Here's how the part is built. I have some questions about the finished solid (model axes, mm). Face numbers are marked on the shaded views. A direction names the side the tool comes from. Round coordinates to 2 decimals unless told otherwise and drop trailing zeros. Write each loop counter-clockwise with the first axis right and the second up, starting at its lowest first coordinate (ties: lowest second). Pieces come first, ordered by that corner, then holes. Notation, with made-up numbers: (73.25, 47) -> (107.25, 47) arc R24 ccw to (107.25, 71) -> close; hole circle Ø11 at (-29, 84.5). An arc over 180 degrees is marked (long way). Answer in a Markdown table with one row per item.
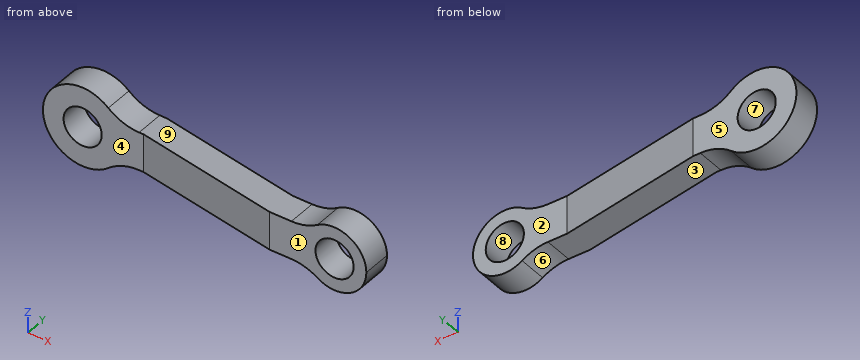
from build123d import *

# Parameters (mm, degrees)
F0_R     = 6
F1_DEPTH = 25
F3_DEPTH = 12.5
F4_R     = 15


with BuildPart() as f1:
    # F0 (on Front) → F1 (new body)
    with BuildSketch(Plane.XZ):
        with BuildLine():
            ThreePointArc((10.965856, -6), (12.110392, -3.096514), (12.5, 0))
            ThreePointArc((12.5, 0), (12.110392, 3.096514), (10.965856, 6))
            ThreePointArc((10.965856, 6), (-12.5, 0), (10.965856, -6))
        make_face()
        Circle(F0_R, mode=Mode.SUBTRACT)
        with BuildLine():
            ThreePointArc((10.965856, 6), (12.110392, 3.096514), (12.5, 0))
            ThreePointArc((12.5, 0), (12.110392, -3.096514), (10.965856, -6))
            Line((10.965856, -6), (77, -6))
            ThreePointArc((77, -6), (75, 0), (77, 6))
            Line((77, 6), (10.965856, 6))
        make_face()
        with BuildLine():
            ThreePointArc((95, 0), (88.162278, 9.486833), (77, 6))
            ThreePointArc((77, 6), (75, 0), (77, -6))
            ThreePointArc((77, -6), (88.162278, -9.486833), (95, 0))
        make_face()
        with Locations((85, 0)):
            Circle(F0_R, mode=Mode.SUBTRACT)
    extrude(amount=F1_DEPTH)

    # F2 (on Top) → F3 (intersect, symmetric)
    with BuildSketch(Plane.XY):
        Polygon((0, 0), (-12.5, 0), (-12.5, -9), (0, -9), (19.212602, -9), (64.582857, -17), (95, -17), (95, -8), (65.370255, -8), (20, 0), align=None)
    extrude(amount=F3_DEPTH, both=True, mode=Mode.INTERSECT)

    # F4
    f4_edges = [f1.edges().sort_by_distance(p)[0] for p in [
        (10.965856, -4.5, -6),
        (10.965856, -4.5, 6),
        (77, -12.5, 6),
        (77, -12.5, -6),
    ]]
    fillet(f4_edges, radius=F4_R)


solid = f1.part
1) I want a section at A-A, the plane x = 85. List the corners of the cut face in (y, z) for me.
Response:
| item | result |
|---|---|
| outline | (-17, -10) -> (-8, -10) -> (-8, -6) -> (-17, -6) -> close; (-17, 6) -> (-8, 6) -> (-8, 10) -> (-17, 10) -> close |
2) For pin 1 (2 mm diameter, centred on y = -11, z = 6, fed in from +X); pin 2 (8 mm diameter, centred on x = 22, y = -15, fed in from -Z); pin 3 (1 mm diameter, centred on x = 36.5, z = 5.5, fed in from +Y); pin 4 (12 mm diameter, centred on x = 13.5, z = 9, fed in from -Y), each with a flat end and sliding along its axis, tell me the tip position at first contact or that it passes through.
Response:
| item | result |
|---|---|
| pin 1 | stops at x = 93.66 |
| pin 2 | passes through |
| pin 3 | stops at y = -2.82 |
| pin 4 | stops at y = -9 |
3) I want a section at B-B, the plane z = -3.75. List the corners of the cut face in (x, y) for me.
Response:
| item | result |
|---|---|
| outline | (-11.92, -9) -> (-4.68, -9) -> (-4.68, 0) -> (-11.92, 0) -> close; (4.68, -9) -> (19.21, -9) -> (64.58, -17) -> (80.32, -17) -> (80.32, -8) -> (65.37, -8) -> (20, 0) -> (4.68, 0) -> close; (89.68, -17) -> (94.27, -17) -> (94.27, -8) -> (89.68, -8) -> close |
4) I want a section at C-C, the plane y = -14.5. List the corners of the cut face in (x, z) for me.
Response:
| item | result |
|---|---|
| outline | (50.4, -6) -> (71.44, -6) arc R15 cw to (79.57, -8.4) arc R10 ccw (long way) to (79.57, 8.4) arc R15 cw to (71.44, 6) -> (50.4, 6) -> close; hole circle Ø12 at (85, 0) |
5) We'd pull the mould along Z, two halves only. Please class the marked faces 6, 7, 8 and 9: +Z half, -Z half, draft (parallel to the pull), parting line (faces both ways), or undercut.
Response:
| item | result |
|---|---|
| face 6 | -Z half |
| face 7 | undercut |
| face 8 | undercut |
| face 9 | +Z half |
6) I want a section at D-D, the plane x = 0. List the corners of the cut face in (y, z) for me.
Response:
| item | result |
|---|---|
| outline | (-9, -12.5) -> (0, -12.5) -> (0, -6) -> (-9, -6) -> close; (-9, 6) -> (0, 6) -> (0, 12.5) -> (-9, 12.5) -> close |
7) Which directions (+Z, -Z, +X, -X, +Y, -Y) give clear straight access to the entire face, cutting with the end or side of a thin tool? Please do the marked faces 1, 2, 3, 4 and 5.
Response:
| item | result |
|---|---|
| face 1 | +Z, -Z, +X, -X, -Y |
| face 2 | +Z, -Z, +X, +Y |
| face 3 | -Z, +Y, -Y |
| face 4 | +Z, -Z, -X, -Y |
| face 5 | +Z, -Z, +X, -X, +Y |
8) I need wall thicknesses on line 1 (Z direction, x = 0, y = -5.25); line 2 (Z direction, x = 85, y = -14); line 3 (X direction, y = -8.25, z = 0). Which ranges of each line are inside material? Lowest first, please. Write a range as [from, to].
Response:
| item | result |
|---|---|
| line 1 | z = [-12.5, -6], [6, 12.5] |
| line 2 | z = [-10, -6], [6, 10] |
| line 3 | x = [-12.5, -6], [6, 79], [91, 95] |
